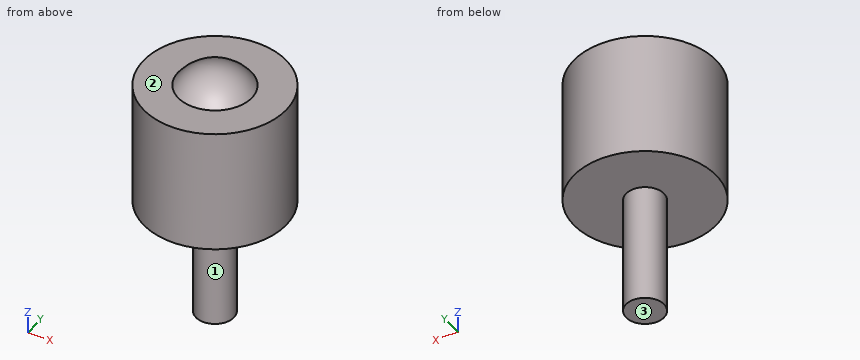
from build123d import *

# Parameters (mm, degrees)
SKETCH3_R           = 4
BOSS_EXTRUDE1_DEPTH = 25


with BuildPart() as part:
    # Sketch1 → Revolve6 (revolve)
    with BuildSketch(Plane(origin=(0, 0, 0), x_dir=(1, 0, 0), z_dir=(0, 1, 0))):
        with BuildLine():
            Line((0, 9.5), (0, -9.5))
            ThreePointArc((0, -9.5), (-9.5, 0), (0, 9.5))
        make_face()
    revolve(axis=Axis((0, 0, -9.5), (0, 0, 1)))

    # Sketch2 → Revolve7 (revolve)
    with BuildSketch(Plane(origin=(0, 0, 0), x_dir=(1, 0, 0), z_dir=(0, 1, 0)), mode=Mode.PRIVATE) as revolve7_sk:
        with BuildLine():
            ThreePointArc((-7.745966692, -5.5), (-9.050875195, -2.886461192), (-9.5, 0))
            Line((-9.5, 0), (-15, 0))
            Line((-15, 0), (-15, -5.5))
            Line((-15, -5.5), (-7.745966692, -5.5))
        make_face()
        with BuildLine():
            Line((-15, 0), (-9.5, 0))
            ThreePointArc((-9.5, 0), (-6.717514421, 6.717514421), (0, 9.5))
            Line((0, 9.5), (0, 20.5))
            Line((0, 20.5), (-15, 20.5))
            Line((-15, 20.5), (-15, 0))
        make_face()
    revolve(revolve7_sk.sketch.rotate(Axis((0, 0, -20.5), (0, 0, 1)), 180), axis=Axis((0, 0, -20.5), (0, 0, 1)))

    # Sketch3 → Boss-Extrude1 (add)
    with BuildSketch(Plane(origin=(0, 0, -20.5), x_dir=(-1, 0, 0), z_dir=(0, 0, -1))):
        Circle(SKETCH3_R)
    extrude(amount=BOSS_EXTRUDE1_DEPTH)


solid = part.part
The listing builds one solid part. Answer for the finished solid, in the listing's coordinates (mm). Face numbers are marked on the shaded views. A direction names the side the tool comes from. Give positions to 0.01 mm unless a question says otherwise; leave off trailing zeros. Order: outer loops, then holes, each group sorted by start corner. A loop starts at its lowest first (then second) coordinate and runs counter-clockwise, first axis right, second up. Notation, with made-up numbers: (0, -28) -> (59, -28) arc R11 cw to (59, -13) -> close; hole circle Ø10 at (-6, 22.5). An arc over 180 degrees is marked (long way). Put each result on its own line as item: value.
Item 1: Straight lines are drawn through the part: line 1 (Z direction, x = 13, y = -2); line 2 (X direction, y = -0.25, z = -20); line 3 (X direction, y = -7.25, z = -9). For each, find the intervals that lie inside material, in ascending order.
Established:
line 1: z = -20.5 to 5.5
line 2: x = -15 to 15
line 3: x = -13.13 to 13.13
Item 2: For the marked faces 1, 2 and 3, determine the directions among +Z, -Z, +X, -X, +Y, -Y from which every point of the face is accessible in a straight line to the end or side of a thin tool.
Established:
face 1: -Z
face 2: +Z
face 3: -Z, +X, -X, +Y, -Y
Item 3: A cutting plane is placed at D-D on z = -1. Give the vertices of the cut face in (x, y).
Established:
outline: circle Ø30 at (0, 0)
Item 4: A cutting plane is placed at C-C on z = -26. Give the vertices of the cut face in (x, y).
Established:
outline: circle Ø8 at (0, 0)
Item 5: Given P1, Ø1.5, axis at x = -4, z = 3.5, coming from the +Y side; P2, Ø9, axis at x = -5, y = 6, coming from the -Z side; P3, Ø4, axis at x = 5, z = -18, coming from the -Y side; P4, Ø9, axis at x = -6, y = 4.5, coming from the +Z side, each flat-ended and moving along its own axis, determine where each tip first touches the part or whether it passes through.
Established:
P1: stops at y = 14.64
P2: stops at z = -45.5
P3: stops at y = -14.7
P4: stops at z = 9.01
Item 6: A cutting plane is placed at A-A on x = 0. Give the vertices of the cut face in (y, z), plus the area to 3 significant figures.
Established:
outline: (-15, -20.5) -> (-4, -20.5) -> (-4, -45.5) -> (4, -45.5) -> (4, -20.5) -> (15, -20.5) -> (15, 5.5) -> (7.75, 5.5) arc R9.5 ccw to (-7.75, 5.5) -> (-15, 5.5) -> close
area: 1,020 mm^2
